Can you work these out from the drawing? Everything is in mm from the part's minimum corner. A direction names the side the tool comes from. Round coordinates to 2 decimals unless told otherwise and drop trailing zeros. Write each loop counter-clockwise with the first axis right and the second up, starting at its lowest first coordinate (ties: lowest second). Pieces come first, ordered by that corner, then holes. Notation, with made-up numbers: M 25,-30 L 39,-30 A19 ccw 39,1 Z; hole C 74,33.25 d6. An arc over 180 degrees is marked long. Answer in a Markdown table with one row per item. Add a question column.
(1) For the marked faces 5, 6 and 7, which set-ups out of +Z, -Z, +X, -X, +Y, -Y let a thin tool reach every point of the face, with its end or its side?
(2) If we mould it in two halves opening along Y, with no side actions, what happens to the marked faces 1, 2, 3 and 4? For each: released by +Y, released by -Y, zero draft, split by the parting line, or undercut.
(3) If I drill on probe 1 along X at (y, z) = (24, 1) (3 decimals); probe 2 along Y at (x, z) = (21.5, 4.5); probe 3 along Y at (x, z) = (11.5, 8.5), over which ranges is the centre line in solid material (lowest first)?
(4) Suppose I cut it at C-C, the plane z = 9.75. Write out the boundary of the cut face in (x, y) (3 decimals).
(5) Suppose I cut it at A-A, the plane y = 4. Write out the boundary of the cut face in (x, z) (3 decimals), then the cut area to 3 significant figures.
(6) Suppose I cut it at D-D, the plane z = 7.39. Write out the boundary of the cut face in (x, y) (3 decimals).
(7) Suppose I cut it at B-B, the plane x = 12. Write out the boundary of the cut face in (y, z), then the cut area to 3 significant figures.
(8) I'm going to push flat-ended pins straight in: pin 1 (3 mm diameter, centred on x = 24, z = 10.5, fed in from +Y); pin 2 (3.5 mm diameter, centred on x = 1, z = 8.5, fed in from +Y); pin 3 (3.5 mm diameter, centred on y = 11, z = 4, fed in from +X) (3 decimals). Where does each tip first touch, or does it pass through?
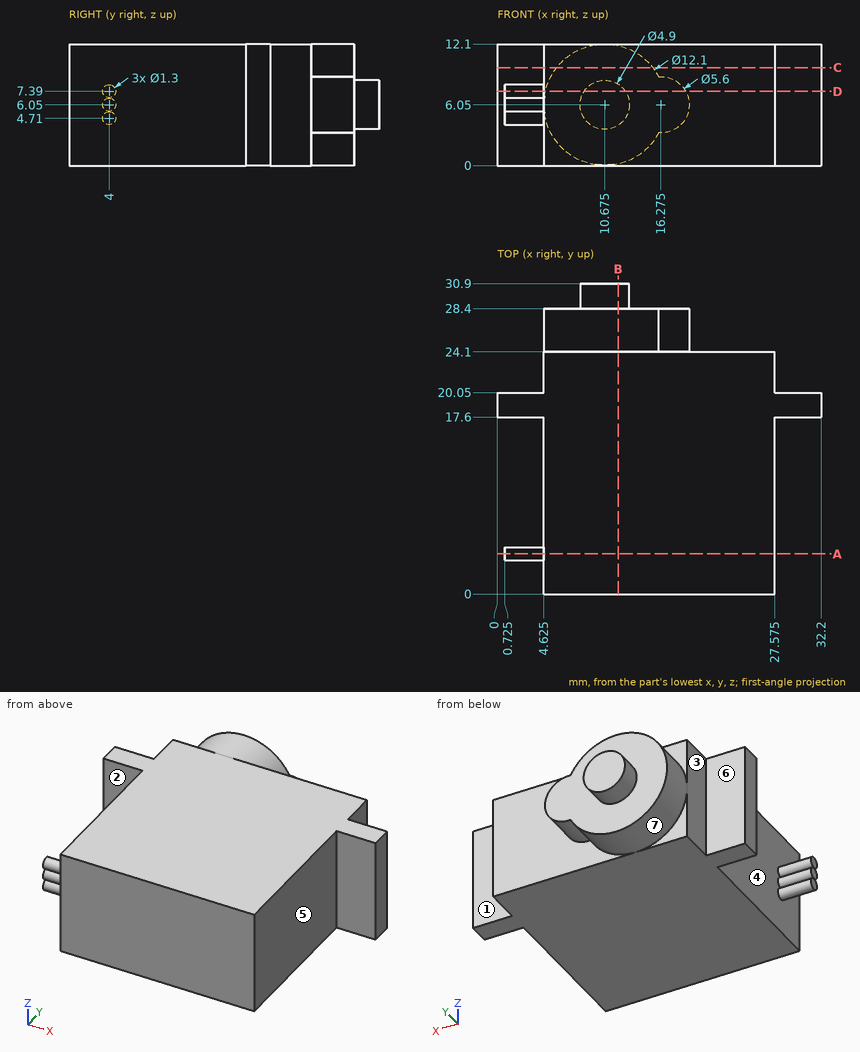
Calculated:
| question | item | result |
|---|---|---|
| 1 | face 5 | +Z, -Z, +X, -Y |
| 1 | face 6 | +Z, -Z, -X, +Y |
| 1 | face 7 | +Y |
| 2 | face 1 | released by +Y |
| 2 | face 2 | undercut |
| 2 | face 3 | zero draft |
| 2 | face 4 | undercut |
| 3 | probe 1 | 4.625 to 27.575 |
| 3 | probe 2 | 0 to 24.1 |
| 3 | probe 3 | 0 to 28.4 |
| 4 | outline | M 0,17.6 L 4.625,17.6 L 4.625,0 L 27.575,0 L 27.575,17.6 L 32.2,17.6 L 32.2,20.05 L 27.575,20.05 L 27.575,24.1 L 15.462,24.1 L 15.462,28.4 L 5.888,28.4 L 5.888,24.1 L 4.625,24.1 L 4.625,20.05 L 0,20.05 Z |
| 5 | outline | M 0.725,4.06 L 4.625,4.06 L 4.625,0 L 27.575,0 L 27.575,12.1 L 4.625,12.1 L 4.625,8.04 L 0.725,8.04 L 0.725,6.74 L 4.625,6.74 L 4.625,6.7 L 0.725,6.7 L 0.725,5.4 L 4.625,5.4 L 4.625,5.36 L 0.725,5.36 Z |
| 5 | area | 293 mm² |
| 6 | outline | M 0,17.6 L 4.625,17.6 L 4.625,4.65 L 0.725,4.65 L 0.725,3.35 L 4.625,3.35 L 4.625,0 L 27.575,0 L 27.575,17.6 L 32.2,17.6 L 32.2,20.05 L 27.575,20.05 L 27.575,24.1 L 18.734,24.1 L 18.734,28.4 L 12.726,28.4 L 12.726,30.9 L 8.624,30.9 L 8.624,28.4 L 4.775,28.4 L 4.775,24.1 L 4.625,24.1 L 4.625,20.05 L 0,20.05 Z |
| 7 | outline | M 0,0 L 24.1,0 L 24.1,0.15 L 28.4,0.15 L 28.4,3.99 L 30.9,3.99 L 30.9,8.11 L 28.4,8.11 L 28.4,11.95 L 24.1,11.95 L 24.1,12.1 L 0,12.1 Z |
| 7 | area | 353 mm² |
| 8 | pin 1 | y = 24.1 |
| 8 | pin 2 | y = 20.05 |
| 8 | pin 3 | x = 27.575 |
